The model under review builds one solid part; all positions refer to its coordinate system, in mm. A direction names the side the tool comes from. Coordinates: 2 decimals unless noted, no trailing zeros. Loops run counter-clockwise (first coordinate to the right, second up) from the corner with the lowest first, then second, coordinate; pieces in that order, holes last. Notation, with made-up numbers: (22, 26.5) - (54, 26.5) arc R27 ccw to (54, 54.5) - close; hole circle Ø6 at (25, 19.5). An arc over 180 degrees is marked (long way). One line per item, written item: value. Start each with the question number.
1. We need section A-A, the plane x = 0. Give the boundary of the cut face in (y, z).
2. Mouldability with a two-part tool opening along Y and no side actions: class faces 1 (the face through (44, -3.175, 3)), 2 (the face through (-44, 3.175, 3)), 3 (the face through (1.9, 0.6, 2.9)) as +Y half, -Y half, draft (parallel to the pull), parting line (faces both ways), or undercut.
3. For faces 4 (the face through (93.06, -1.72, 2.86)), 5 (the face through (-45, -3.175, 3)), 6 (the face through (45, 3.175, 3)), list the 3-axis set-ups (+Z, -Z, +X, -X, +Y, -Y) from which the entire face can be reached by the end or side of a thin tool; tool diameter is ignored.
4. We need section D-D, the plane x = 88.9. Give the boundary of the cut face in (y, z).
5. To check wall thickness, follow line 1 (Y direction, x = 88.9, z = 4.15); line 2 (X direction, y = -3.75, z = 4.65); line 3 (X direction, y = -0.25, z = 0.95). State the ranges of each line that lie inside material, in increasing order.
6. Insertion check: P1, Ø3, axis at x = -26, z = 3, coming from the -Y side (3 decimals); P2, Ø1, axis at x = 59, z = 1.5, coming from the +Y side (3 decimals). Each pin has a flat end and moves straight along its axis. Give the tip position at first contact, or say it passes through.
7. We need section B-B, the plane y = 0. Give the boundary of the cut face in (x, z).
8. We need section C-C, the plane z = 2.35. Give the boundary of the cut face in (x, y) (3 decimals), then the cut area to 3 significant figures.
from build123d import *

# Parameters (mm, degrees)
SKETCH1_R           = 4.49961
SKETCH1_R_2         = 1.9939
BOSS_EXTRUDE1_DEPTH = 5.80136
FILLET1_R           = 3.175


with BuildPart() as part:
    # Sketch1 → Boss-Extrude1 (new body)
    with BuildSketch(Plane.XY):
        with BuildLine():
            Line((-83.400738686, -3.175), (-5.499261314, -3.175))
            ThreePointArc((-5.499261314, -3.175), (0, -6.35), (5.499261314, -3.175))
            Line((5.499261314, -3.175), (83.400738686, -3.175))
            ThreePointArc((83.400738686, -3.175), (95.25, 0), (83.400738686, 3.175))
            Line((83.400738686, 3.175), (5.499261314, 3.175))
            ThreePointArc((5.499261314, 3.175), (0, 6.35), (-5.499261314, 3.175))
            Line((-5.499261314, 3.175), (-83.400738686, 3.175))
            ThreePointArc((-83.400738686, 3.175), (-95.25, 0), (-83.400738686, -3.175))
        make_face()
        with Locations((-88.9, 0)):
            Circle(SKETCH1_R, mode=Mode.SUBTRACT)
        Circle(SKETCH1_R_2, mode=Mode.SUBTRACT)
        with Locations((88.9, 0)):
            Circle(SKETCH1_R, mode=Mode.SUBTRACT)
    extrude(amount=BOSS_EXTRUDE1_DEPTH)

    # Fillet1
    fillet1_edges = [part.edges().sort_by_distance(p)[0] for p in [
        (-83.400738686, 3.175, 2.90068),
        (-5.499261314, 3.175, 2.90068),
        (5.499261314, 3.175, 2.90068),
        (83.400738686, 3.175, 2.90068),
        (83.400738686, -3.175, 2.90068),
        (5.499261314, -3.175, 2.90068),
        (-5.499261314, -3.175, 2.90068),
        (-83.400738686, -3.175, 2.90068),
    ]]
    fillet(fillet1_edges, radius=FILLET1_R)


solid = part.part
Findings below:
1. outline: (-6.35, 0) - (-1.99, 0) - (-1.99, 5.8) - (-6.35, 5.8) - close; (1.99, 0) - (6.35, 0) - (6.35, 5.8) - (1.99, 5.8) - close
2. face 1: -Y half
2. face 2: +Y half
2. face 3: undercut
3. face 4: +Z, -Z
3. face 5: +Z, -Z, -Y
3. face 6: +Z, -Z, +Y
4. outline: (-6.35, 0) - (-4.5, 0) - (-4.5, 5.8) - (-6.35, 5.8) - close; (4.5, 0) - (6.35, 0) - (6.35, 5.8) - (4.5, 5.8) - close
5. line 1: -6.35 to -4.5, 4.5 to 6.35
5. line 2: -94.02 to -91.39, -86.41 to -83.62, -5.28 to 5.28, 83.62 to 86.41, 91.39 to 94.02
5. line 3: -95.25 to -93.39, -84.41 to -1.98, 1.98 to 84.41, 93.39 to 95.25
6. P1: y = -3.175
6. P2: y = 3.175
7. outline: (-95.25, 0) - (-93.4, 0) - (-93.4, 5.8) - (-95.25, 5.8) - close; (-84.4, 0) - (-1.99, 0) - (-1.99, 5.8) - (-84.4, 5.8) - close; (1.99, 0) - (84.4, 0) - (84.4, 5.8) - (1.99, 5.8) - close; (93.4, 0) - (95.25, 0) - (95.25, 5.8) - (93.4, 5.8) - close
8. outline: (-84.167, -4.233) arc R3.175 cw to (-81.8, -3.175) - (-7.1, -3.175) arc R3.175 cw to (-4.733, -4.233) arc R6.35 ccw to (4.733, -4.233) arc R3.175 cw to (7.1, -3.175) - (81.8, -3.175) arc R3.175 cw to (84.167, -4.233) arc R6.35 ccw (long way) to (84.167, 4.233) arc R3.175 cw to (81.8, 3.175) - (7.1, 3.175) arc R3.175 cw to (4.733, 4.233) arc R6.35 ccw to (-4.733, 4.233) arc R3.175 cw to (-7.1, 3.175) - (-81.8, 3.175) arc R3.175 cw to (-84.167, 4.233) arc R6.35 ccw (long way) to start; hole circle Ø8.999 at (-88.9, 0); hole circle Ø3.988 at (0, 0); hole circle Ø8.999 at (88.9, 0)
8. area: 1,220 mm2
